Can you work these out from the model? Positions are in its coordinate system, mm. A direction names the side the tool comes from. Coordinates: 2 decimals unless noted, no trailing zeros. Loops run counter-clockwise (first coordinate to the right, second up) from the corner with the lowest first, then second, coordinate; pieces in that order, holes last.
```python
from build123d import *

# Parameters (mm, degrees)
BOSS_EXTRUDE1_DEPTH = 549.91
SKETCH2_R           = 9
CUT_EXTRUDE1_DEPTH  = 10
CUT_EXTRUDE2_DEPTH  = 10


with BuildPart() as part:
    # Sketch1 → Boss-Extrude1 (new body)
    with BuildSketch(Plane.XY):
        Polygon((-9.285714286, 23.80952381), (-9.285714286, -26.19047619), (25.714285714, -26.19047619), (25.714285714, -21.19047619), (-4.285714286, -21.19047619), (-4.285714286, 23.80952381), align=None)
    extrude(amount=BOSS_EXTRUDE1_DEPTH)

    # Sketch2 → Cut-Extrude1 (cut)
    with BuildSketch(Plane(origin=(-4.285714286, 0, 0), x_dir=(0, 0, -1), z_dir=(1, 0, 0))):
        with Locations(Location((-524.91, 1.249990258, 0), (0, 0, 90))):
            Circle(SKETCH2_R)
        with Locations(Location((-485, 1.154950897, 0), (0, 0, 90))):
            Circle(SKETCH2_R)
        with Locations(Location((-64.91, 0.154572913, 0), (0, 0, 90))):
            Circle(SKETCH2_R)
        with Locations(Location((-25, 0.059533551, 0), (0, 0, 90))):
            Circle(SKETCH2_R)
    extrude(amount=-CUT_EXTRUDE1_DEPTH, mode=Mode.SUBTRACT)

    # Sketch3 → Cut-Extrude2 (cut)
    with BuildSketch(Plane(origin=(0, -21.19047619, 0), x_dir=(1, 0, 0), z_dir=(0, 1, 0))):
        with BuildLine():
            Line((1.733492456, -360.884266397), (1.697419827, -336.465805265))
            ThreePointArc((1.697419827, -336.465805265), (10.6962494, -327.610947677), (19.695078973, -336.465805265))
            Line((19.695078973, -336.465805265), (19.733492456, -360.884266397))
            ThreePointArc((19.733492456, -360.884266397), (10.733492456, -369.884266397), (1.733492456, -360.884266397))
        make_face()
        with BuildLine():
            Line((1.582473361, -247.923607511), (1.546400733, -223.505146379))
            ThreePointArc((1.546400733, -223.505146379), (10.545230305, -214.650288791), (19.544059878, -223.505146379))
            Line((19.544059878, -223.505146379), (19.582473361, -247.923607511))
            ThreePointArc((19.582473361, -247.923607511), (10.582473361, -256.923607511), (1.582473361, -247.923607511))
        make_face()
    extrude(amount=-CUT_EXTRUDE2_DEPTH, mode=Mode.SUBTRACT)


solid = part.part
```
(1) I want a section at A-A on z = 25. Write out the boundary of the cut face in (x, y).
Check values:
outline: (-9.29, -26.19) - (25.71, -26.19) - (25.71, -21.19) - (-4.29, -21.19) - (-4.29, -8.94) - (-9.29, -8.94) - close; (-9.29, 9.06) - (-4.29, 9.06) - (-4.29, 23.81) - (-9.29, 23.81) - close
(2) If I drill on probe 1 along Z at (x, y) = (-5.5, 0); probe 2 along Z at (x, y) = (-5, -0.5); probe 3 along X at (y, z) = (-18, 206.5), over which ranges is the centre line in solid material (lowest first)?
Check values:
probe 1: z = 0 to 16, 34 to 55.91, 73.91 to 476.07, 493.93 to 516, 533.82 to 549.91
probe 2: z = 0 to 16.02, 33.98 to 55.93, 73.89 to 476.15, 493.85 to 516.08, 533.74 to 549.91
probe 3: x = -9.29 to -4.29
(3) If we mould it in two halves opening along Y, with no side actions, what happens to faces 4 (the flat face through (-4.286, 1, 271)), 5 (the cylindrical face through (-6.75, 4.99, 72.5)), 6 (the flat face through (8, -26.19, 271)), 7 (the cylindrical face through (-6.751, 0.078, 533.833))? For each: released by +Y, released by -Y, zero draft, split by the parting line, or undercut.
Check values:
face 4: zero draft
face 5: undercut
face 6: released by -Y
face 7: undercut
(4) I want a section at B-B on y = -2. Write out the boundary of the cut face in (x, z).
Check values:
outline: (-9.29, 0) - (-4.29, 0) - (-4.29, 16.24) - (-9.29, 16.24) - close; (-9.29, 33.76) - (-4.29, 33.76) - (-4.29, 56.17) - (-9.29, 56.17) - close; (-9.29, 73.65) - (-4.29, 73.65) - (-4.29, 476.57) - (-9.29, 476.57) - close; (-9.29, 493.43) - (-4.29, 493.43) - (-4.29, 516.52) - (-9.29, 516.52) - close; (-9.29, 533.3) - (-4.29, 533.3) - (-4.29, 549.91) - (-9.29, 549.91) - close
(5) I want a section at C-C on z = 234. Write out the boundary of the cut face in (x, y), then the cut area to 3 significant figures.
Check values:
outline: (-9.29, -26.19) - (1.56, -26.19) - (1.56, -21.19) - (-4.29, -21.19) - (-4.29, 23.81) - (-9.29, 23.81) - close; (19.56, -26.19) - (25.71, -26.19) - (25.71, -21.19) - (19.56, -21.19) - close
area: 310 mm2
(6) Which directions (+Z, -Z, +X, -X, +Y, -Y) give clear straight access to the entire face, cutting with the end or side of a thin tool? Please do faces 1 (the flat face through (11, -21.19, 271)), 2 (the cylindrical face through (-6.751, 8.644, 27.703)), 3 (the cylindrical face through (10.78, -23.66, 256.92)).
Check values:
face 1: +Z, -Z, +X, +Y
face 2: +X, -X
face 3: +Y, -Y
(7) I'm going to push flat-ended pins straight in: pin 1 (23.5 mm diameter, centred on y = 0.15, z = 64.91, fed in from +X); pin 2 (4 mm diameter, centred on x = 11.5, z = 266.5, fed in from +Y). Where does each tip first touch, or does it pass through?
Check values:
pin 1: stops at x = -4.29
pin 2: stops at y = -21.19
